Build history of the part. All positions in model axes, mm. Give positions to 0.01 mm unless a question says otherwise; leave off trailing zeros. Write each loop counter-clockwise with the first axis right and the second up, starting at its lowest first coordinate (ties: lowest second). Pieces come first, ordered by that corner, then holes. Notation, with made-up numbers: (30, 1) -> (61, 1) arc R11 cw to (61, 20) -> close; hole circle Ø10 at (-28, 30.5). An arc over 180 degrees is marked (long way). Put each result on its own line as item: value. Start each with the question number.
Item 1: Slice it at B-B, the plane z = 0. List the corners of the cut face in (x, y).
Item 2: Drill centre lines: line 1 along X through (y, z) = (0.1, -0.05); line 2 along Z through (x, y) = (13.5, 0.45). Where is each one in solid material? Low to high.
Item 3: Slice it at A-A, the plane x = -13.5. List the corners of the cut face in (y, z).
Item 4: Slice it at C-C, the plane y = 0.2. List the corners of the cut face in (x, z).
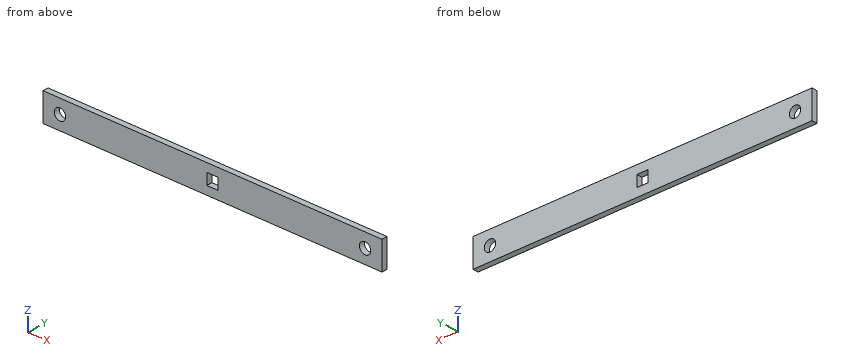
```python
from build123d import *

# Parameters (mm, degrees)
SKETCH2_W               = 30
SKETCH2_H               = 2.5
BOSS_EXTRUDE1_DEPTH     = 0.5
CUT_EXTRUDE1_DEPTH      = 16.060295482
CUT_EXTRUDE1_DEPTH_BACK = 16.060295482
SKETCH3_R               = 0.5
SKETCH3_W               = 1
SKETCH3_H               = 1


with BuildPart() as part:
    # Sketch2 → Boss-Extrude1 (new body)
    with BuildSketch(Plane(origin=(0, 0, 0), x_dir=(1, 0, 0), z_dir=(0, 1, 0))):
        Rectangle(SKETCH2_W, SKETCH2_H)
    extrude(amount=BOSS_EXTRUDE1_DEPTH)

    # Sketch3 → Cut-Extrude1 (cut, two sides: drawn at the far end of the back side and taken through both)
    with BuildSketch(Plane(origin=(0, 0.5, 0), x_dir=(1, 0, 0), z_dir=(0, 1, 0)).offset(-CUT_EXTRUDE1_DEPTH_BACK)):
        with Locations(Location((-13.5, 0, 0), (0, 0, 270))):
            Circle(SKETCH3_R)
        with Locations(Location((13.5, 0, 0), (0, 0, 270))):
            Circle(SKETCH3_R)
        Rectangle(SKETCH3_W, SKETCH3_H)
    extrude(amount=CUT_EXTRUDE1_DEPTH + CUT_EXTRUDE1_DEPTH_BACK, mode=Mode.SUBTRACT)


solid = part.part
```
Values follow:
1. outline: (-15, 0) -> (-14, 0) -> (-14, 0.5) -> (-15, 0.5) -> close; (-13, 0) -> (-0.5, 0) -> (-0.5, 0.5) -> (-13, 0.5) -> close; (0.5, 0) -> (13, 0) -> (13, 0.5) -> (0.5, 0.5) -> close; (14, 0) -> (15, 0) -> (15, 0.5) -> (14, 0.5) -> close
2. line 1: -15 to -14, -13 to -0.5, 0.5 to 13, 14 to 15
2. line 2: -1.25 to -0.5, 0.5 to 1.25
3. outline: (0, -1.25) -> (0.5, -1.25) -> (0.5, -0.5) -> (0, -0.5) -> close; (0, 0.5) -> (0.5, 0.5) -> (0.5, 1.25) -> (0, 1.25) -> close
4. outline: (-15, -1.25) -> (15, -1.25) -> (15, 1.25) -> (-15, 1.25) -> close; hole circle Ø1 at (-13.5, 0); hole (-0.5, -0.5) -> (0.5, -0.5) -> (0.5, 0.5) -> (-0.5, 0.5) -> close; hole circle Ø1 at (13.5, 0)
